from build123d import *

# Parameters (mm, degrees)
F0_R     = 45
F1_DEPTH = 13
F3_DEPTH = 16
F4_R     = 2.2
F5_DEPTH = 14


with BuildPart() as f1:
    # F0 (on Top) → F1 (new body)
    with BuildSketch(Plane.XY):
        Circle(F0_R)
    extrude(amount=F1_DEPTH)

    # F2 (on face) → F3 (cut)
    with BuildSketch(Plane.XY.offset(13)):
        with BuildLine():
            Line((2.833725, 3.1), (-2.833725, 3.1))
            ThreePointArc((-2.833725, 3.1), (0, -4.2), (2.833725, 3.1))
        make_face()
    extrude(amount=-F3_DEPTH, mode=Mode.SUBTRACT)

    # F4 (on face) → F5 (cut)
    with BuildSketch(Plane.XY.offset(13)):
        with Locations((0, 35)):
            Circle(F4_R)
        with Locations((35, 0)):
            Circle(F4_R)
        with Locations((-35, 0)):
            Circle(F4_R)
        with Locations((0, -35)):
            Circle(F4_R)
    extrude(amount=-F5_DEPTH, mode=Mode.SUBTRACT)


solid = f1.part
Could you check a few things on this model? Use its own coordinates, in mm. A direction names the side the tool comes from. Give positions to 0.01 mm unless a question says otherwise; leave off trailing zeros. Order: outer loops, then holes, each group sorted by start corner. A loop starts at its lowest first (then second) coordinate and runs counter-clockwise, first axis right, second up.
1. Suppose I cut it at B-B (y = 0). List the corners of the cut face in (x, z) for me.
2. Will these pins go through, and if not, where does the flat tip stop? P1, Ø6, axis at y = 29.5, z = 4, coming from the +X side; P2, Ø6, axis at y = -10, z = 2.5, coming from the -X side; P3, Ø4, axis at x = 21.5, y = -10, coming from the -Z side; P4, Ø2, axis at x = -25, z = 5, coming from the -Y side.
3. For faces 1 (the flat face through (-1, -9, 0)), 2 (the flat face through (0, 3.1, 7)), which set-ups out of +Z, -Z, +X, -X, +Y, -Y let a thin tool reach every point of the face, with its end or its side?
4. I need wall thicknesses on L1, parallel to Y at x = 0, z = 3.75; L2, parallel to Y at x = -35, z = 7.25; L3, parallel to X at y = 33, z = 9.25. Which ranges of each line are inside material? Lowest first, please.
5. Suppose I cut it at A-A (x = 0). List the corners of the cut face in (y, z) for me, plus the area to 3 significant figures.
6. Suppose I cut it at D-D (y = 35). List the corners of the cut face in (x, z) for me, plus the area to 3 significant figures.
7. Suppose I cut it at C-C (z = 5.25). List the corners of the cut face in (x, y) for me.
Solved:
1. outline: (-45, 0) - (-37.2, 0) - (-37.2, 13) - (-45, 13) - close; (-32.8, 0) - (-4.2, 0) - (-4.2, 13) - (-32.8, 13) - close; (4.2, 0) - (32.8, 0) - (32.8, 13) - (4.2, 13) - close; (37.2, 0) - (45, 0) - (45, 13) - (37.2, 13) - close
2. P1: stops at x = 36.37
2. P2: stops at x = -44.45
2. P3: stops at z = 0
2. P4: stops at y = -38.07
3. face 1: -Z, +X, -X, +Y, -Y
3. face 2: +Z, -Z
4. L1: y = -45 to -37.2, -32.8 to -4.2, 3.1 to 32.8, 37.2 to 45
4. L2: y = -28.28 to -2.2, 2.2 to 28.28
4. L3: x = -30.59 to -0.92, 0.92 to 30.59
5. outline: (-45, 0) - (-37.2, 0) - (-37.2, 13) - (-45, 13) - close; (-32.8, 0) - (-4.2, 0) - (-4.2, 13) - (-32.8, 13) - close; (3.1, 0) - (32.8, 0) - (32.8, 13) - (3.1, 13) - close; (37.2, 0) - (45, 0) - (45, 13) - (37.2, 13) - close
5. area: 961 mm2
6. outline: (-28.28, 0) - (-2.2, 0) - (-2.2, 13) - (-28.28, 13) - close; (2.2, 0) - (28.28, 0) - (28.28, 13) - (2.2, 13) - close
6. area: 678 mm2
7. outline: circle Ø90 at (0, 0); hole circle Ø4.4 at (-35, 0); hole (-2.83, 3.1) arc R4.2 ccw (long way) to (2.83, 3.1) - close; hole circle Ø4.4 at (0, -35); hole circle Ø4.4 at (0, 35); hole circle Ø4.4 at (35, 0)
